Check sheet for the modelled part. Datum: model origin and axes. Units: mm. A direction names the side the tool comes from. Give positions to 0.01 mm unless a question says otherwise; leave off trailing zeros. Write each loop counter-clockwise with the first axis right and the second up, starting at its lowest first coordinate (ties: lowest second). Pieces come first, ordered by that corner, then holes. Notation, with made-up numbers: M 79,-6.75 L 129,-6.75 A15 ccw 129,-1.75 Z; hole C -38.5,-33.75 d8. An arc over 180 degrees is marked long. Write item = value, one per line. Start each with the question number.
1) Draft check along X on faces 1 (the face through (-10.889, 23.94, -34.576)), 2 (the face through (1, 0, -1)), 3 (the face through (-20.796, 3.844, 21.148)). Enter one of: pulls with the +X half, pulls with the -X half, needs draft (parallel to the pull), parting line crosses it, or undercut.
2) Gauge pin test, flat ends, axial feed: pin 1 (12 mm diameter, centred on x = -3.5, z = -33.5, fed in from -Y); pin 2 (6 mm diameter, centred on x = -1, y = 29, fed in from +Z); pin 3 (0.9 mm diameter, centred on x = 0.5, z = -39.5, fed in from -Y); pin 4 (6 mm diameter, centred on x = 20.5, y = 4, fed in from +Z). Record the tip position at first contact, or that the pin passes through.
3) Sectioned sample at B-B, the plane x = 0. Record the cut outline in (y, z).
4) Sectioned sample at A-A, the plane z = 0. Record the cut outline in (x, y).
5) Scan lines: L1, parallel to X at y = 7.5, z = -50; L2, parallel to Y at x = -10.5, z = 24; L3, parallel to Y at x = -0.5, z = -32. Record each from-to range of solid material in increasing order.
6) Set-up check for faces 4 (the face through (5.5, 5.6, -39.7)), 5 (the face through (0, 8, -52)), 6 (the face through (0, 1.5, -40)), 7 (the face through (21.64, 1.52, -19.35)): record each of +Z, -Z, +X, -X, +Y, -Y from which the full face is reachable in a straight line by a thin tool's end or side.
7) Sectioned sample at D-D, the plane y = 11.5. Record the cut outline in (x, z), then the cut area to 3 significant figures.
8) Sectioned sample at C-C, the plane y = 5.5. Record the cut outline in (x, z), then the cut area to 3 significant figures.
from build123d import *

# Parameters (mm, degrees)
ESQUISSE1_R                         = 37.85
BOSS_EXTRU_1_DEPTH                  = 18.6
ENL_V_MAT_EXTRU_1_DEPTH             = 20
D_GAGEMENT_M31_D                    = 3.4
D_GAGEMENT_M31_DEPTH                = 3
D_GAGEMENT_M31_TIP                  = 1.021463052
BOSS_EXTRU_2_DEPTH                  = 4
BOSS_EXTRU_2_DIRECTION_2_REACH      = 96.043
BOSS_EXTRU_2_DIRECTION_2_END_RADIUS = 37.85
ESQUISSE9_R                         = 2.5
BOSS_EXTRU_3_DEPTH                  = 20


with BuildPart() as part:
    # Esquisse1 → Boss.-Extru.1 (new body)
    with BuildSketch(Plane(origin=(0, 0, 0), x_dir=(1, 0, 0), z_dir=(0, 1, 0))):
        with Locations(Location((0, 0, 0), (0, 0, 270))):
            Circle(ESQUISSE1_R)
    extrude(amount=BOSS_EXTRU_1_DEPTH)

    # Esquisse2 → Révolution1 (revolve)
    with BuildSketch(Plane.XY, mode=Mode.PRIVATE) as r_volution1_sk:
        with BuildLine():
            Line((0, 18.6), (0, 41))
            Line((0, 41), (-24.682338214, 41))
            ThreePointArc((-24.682338214, 41), (-32.861910305, 37.611910305), (-36.25, 29.432338214))
            Line((-36.25, 29.432338214), (-36.25, 18.6))
            Line((-36.25, 18.6), (0, 18.6))
        make_face()
    revolve(r_volution1_sk.sketch.rotate(Axis((0, 18.6, 0), (0, 1, 0)), 270), axis=Axis((0, 18.6, 0), (0, 1, 0)))

    # Esquisse3 → Enlèv. mat.-Extru.1 (cut)
    with BuildSketch(Plane.XY.offset(36.25)):
        with BuildLine():
            Line((-20, 37), (20, 37))
            ThreePointArc((20, 37), (26, 31), (20, 25))
            Line((20, 25), (-20, 25))
            ThreePointArc((-20, 25), (-26, 31), (-20, 37))
        make_face()
    extrude(amount=-ENL_V_MAT_EXTRU_1_DEPTH, mode=Mode.SUBTRACT)

    # Dégagement M31
    with Locations(Plane(origin=(0, 0, 0), x_dir=(-1, 0, 0), z_dir=(0, -1, 0))):
        with Locations((20.859650045, -20.859650045), (-20.859650045, -20.859650045), (-20.859650045, 20.859650045), (20.859650045, 20.859650045)):
            Hole(D_GAGEMENT_M31_D / 2, depth=D_GAGEMENT_M31_DEPTH)
            with Locations((0, 0, -(D_GAGEMENT_M31_DEPTH + D_GAGEMENT_M31_TIP / 2))):  # 118° drill point
                Cone(0, D_GAGEMENT_M31_D / 2, D_GAGEMENT_M31_TIP, mode=Mode.SUBTRACT)

    # Esquisse8 → Boss.-Extru.2 (add)
    with BuildSketch(Plane.XY.offset(-37.85)):
        with BuildLine():
            Line((-1.5, 9.5), (1.5, 9.5))
            ThreePointArc((1.5, 9.5), (5.5, 5.5), (1.5, 1.5))
            Line((1.5, 1.5), (-1.5, 1.5))
            ThreePointArc((-1.5, 1.5), (-5.5, 5.5), (-1.5, 9.5))
        make_face()
    extrude(amount=-BOSS_EXTRU_2_DEPTH)

    # Boss.-Extru.2 direction 2: up to this cylinder (the profile starts outside it)
    boss_extru_2_direction_2_end = Plane(origin=(0, 5.5, 0), z_dir=(0, -1, 0)) * Cylinder(BOSS_EXTRU_2_DIRECTION_2_END_RADIUS, 268.786, mode=Mode.PRIVATE)
    # Esquisse8 → Boss.-Extru.2 direction 2 (add, up to the surface)
    with BuildSketch(Plane.XY.offset(-37.85), mode=Mode.PRIVATE) as boss_extru_2_direction_2_sk1:
        with BuildLine():
            Line((-1.5, 9.5), (1.5, 9.5))
            ThreePointArc((1.5, 9.5), (5.5, 5.5), (1.5, 1.5))
            Line((1.5, 1.5), (-1.5, 1.5))
            ThreePointArc((-1.5, 1.5), (-5.5, 5.5), (-1.5, 9.5))
        make_face()
    boss_extru_2_direction_2_tool1 = extrude(boss_extru_2_direction_2_sk1.sketch, amount=BOSS_EXTRU_2_DIRECTION_2_REACH, mode=Mode.PRIVATE) - boss_extru_2_direction_2_end
    add(boss_extru_2_direction_2_tool1.solids().sort_by_distance((0, 5.5, -37.85))[0])
    add(boss_extru_2_direction_2_tool1.solids().sort_by_distance((0, 5.5, -37.85))[1])

    # Esquisse9 → Boss.-Extru.3 (add)
    with BuildSketch(Plane(origin=(0, 0, -41.85), x_dir=(-1, 0, 0), z_dir=(0, 0, -1))):
        with Locations((0, 5.5)):
            Circle(ESQUISSE9_R)
    extrude(amount=BOSS_EXTRU_3_DEPTH)


solid = part.part
Data:
q1.face_1 = parting line crosses it
q1.face_2 = needs draft
q1.face_3 = undercut
q2.pin_1 = 0
q2.pin_2 = 16.25
q2.pin_3 = 1.5
q2.pin_4 = 33.56
q3.outline = M 0,-37.85 L 1.5,-37.85 L 1.5,-41.85 L 3,-41.85 L 3,-61.85 L 8,-61.85 L 8,-41.85 L 9.5,-41.85 L 9.5,-37.85 L 18.6,-37.85 L 18.6,-36.25 L 29.43,-36.25 A11.57 ccw 41,-24.68 L 41,24.68 A11.57 ccw 37,33.43 L 37,16.25 L 25,16.25 L 25,36.25 L 18.6,36.25 L 18.6,37.85 L 0,37.85 Z
q4.outline = M -37.85,0 L 37.85,0 L 37.85,18.6 L 36.25,18.6 L 36.25,29.43 A11.57 ccw 24.68,41 L -24.68,41 A11.57 ccw -36.25,29.43 L -36.25,18.6 L -37.85,18.6 Z
q5.L1 = -1.5 to 1.5
q5.L2 = 0 to 25, 37 to 40.9
q5.L3 = 0 to 38.39
q6.face_4 = -Z, +X
q6.face_5 = -Z
q6.face_6 = -Z, +X, -X, -Y
q6.face_7 = -Y
q7.outline = C 0,0 d75.7
q7.area = 4,500 mm2
q8.outline = M -5.5,-41.85 L -2.5,-41.85 L -2.5,-61.85 L 2.5,-61.85 L 2.5,-41.85 L 5.5,-41.85 L 5.5,-37.45 A37.85 ccw long -5.5,-37.45 Z
q8.area = 4,650 mm2
